Geometry: final body of the model. Coordinates: model frame, mm. Round coordinates to 2 decimals unless told otherwise and drop trailing zeros. Loops run counter-clockwise (first coordinate to the right, second up) from the corner with the lowest first, then second, coordinate; pieces in that order, holes last. Notation, with made-up numbers: (89.5, -39.5) - (101.5, -39.5) arc R13 ccw to (101.5, -23.5) - close; hole circle Ø10 at (89.5, 14.25). An arc over 180 degrees is marked (long way). Use CSV: the item, a comma, the result in double quotes.
from build123d import *

# Parameters (mm, degrees)
SKETCH1_R           = 0.25
BOSS_EXTRUDE1_DEPTH = 2
SWEEP1_OUTLINE_R    = 0.25
SWEEP1_DEPTH        = 2.5
SWEEP1_2_OUTLINE_R  = 0.25
SWEEP1_2_ANGLE      = 90
SWEEP1_3_OUTLINE_R  = 0.25
SWEEP1_3_ANGLE      = 90
SWEEP1_START        = 0.4999999
SWEEP1_4_OUTLINE_R  = 0.25
SWEEP1_4_DEPTH      = 40.9000002


with BuildPart() as part:
    # Sketch1 → Boss-Extrude1 (new body)
    with BuildSketch(Plane(origin=(0, 0, 0), x_dir=(1, 0, 0), z_dir=(0, 1, 0))):
        with Locations(Location((0, 0, 0), (0, 0, 270))):
            Circle(SKETCH1_R)
    extrude(amount=BOSS_EXTRUDE1_DEPTH)

    # Sweep1: read off the stored shape, not the designer's step
    # Sweep1 outline → Sweep1 (add)
    with BuildSketch(Plane(origin=(0, 0, 0), x_dir=(1, 0, 0), z_dir=(0, 1, 0))):
        Circle(SWEEP1_OUTLINE_R)
        with Locations((41.9, 0)):
            Circle(SWEEP1_OUTLINE_R)
    extrude(amount=SWEEP1_DEPTH)

    # Sweep1 2 outline → Sweep1 2 (revolve)
    with BuildSketch(Plane(origin=(0.5, 2.5, 0), x_dir=(0, 1, 0), z_dir=(1, 0, 0))):
        with Locations((0.5, 0)):
            Circle(SWEEP1_2_OUTLINE_R)
    revolve(axis=Axis((0.5, 2.5, 0), (0, 0, 1)), revolution_arc=SWEEP1_2_ANGLE)

    # Sweep1 3 outline → Sweep1 3 (revolve)
    with BuildSketch(Plane(origin=(41.4, 2.5, 0), x_dir=(1, 0, 0), z_dir=(0, -1, 0))):
        with Locations((0.5, 0)):
            Circle(SWEEP1_3_OUTLINE_R)
    revolve(axis=Axis((41.4, 2.5, 0), (0, 0, 1)), revolution_arc=SWEEP1_3_ANGLE)

    # Sweep1 4 outline → Sweep1 4 (add)
    with BuildSketch(Plane.YZ.offset(SWEEP1_START)):
        with Locations((3, 0)):
            Circle(SWEEP1_4_OUTLINE_R)
    extrude(amount=SWEEP1_4_DEPTH)


solid = part.part
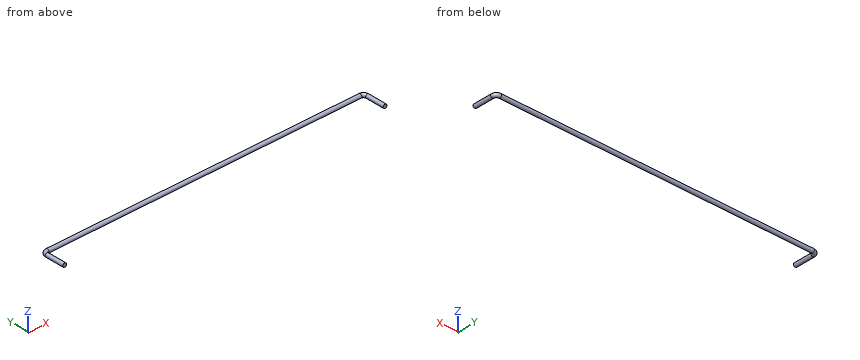
Item 1: Section C-C on x = 26. Return the cut outline in (y, z).
Final values:
outline,"circle Ø0.5 at (3, 0)"
Item 2: Section A-A on y = 0.4. Return the cut outline in (x, z), plus the area to 3 significant figures.
Final values:
outline,"circle Ø0.5 at (0, 0); circle Ø0.5 at (41.9, 0)"
area,"0.393 mm²"
Item 3: Section B-B on z = 0.15. Return the cut outline in (x, y).
Final values:
outline,"(-0.2, 0) - (0.2, 0) - (0.2, 2.5) arc R0.3 cw to (0.5, 2.8) - (41.4, 2.8) arc R0.3 cw to (41.7, 2.5) - (41.7, 0) - (42.1, 0) - (42.1, 2.5) arc R0.7 ccw to (41.4, 3.2) - (0.5, 3.2) arc R0.7 ccw to (-0.2, 2.5) - close"
Item 4: Material intervals for line 1 (X direction, y = 2.45, z = 0.05); line 2 (Y direction, x = 4, z = 0.05); line 3 (X direction, y = 2.55, z = -0.2), sorted ascending.
Final values:
line 1,"x = -0.24 to 0.24, 41.66 to 42.14"
line 2,"y = 2.76 to 3.24"
line 3,"x = -0.15 to 0.15, 41.75 to 42.05"
